```python
from build123d import *

# Parameters (mm, degrees)
EXTRUDE_THIN3_DEPTH     = 70
CUT_EXTRUDE1_DEPTH      = 76.511321578
CUT_EXTRUDE1_DEPTH_BACK = 76.511321578
SKETCH9_R               = 4.064
CUT_EXTRUDE2_DEPTH      = 2.54
LPATTERN1_COUNT         = 2
LPATTERN1_PITCH         = 12.7


# Read off the part's stored shape, not the designer's step: Mirror1
with BuildPart() as part:
    # Sketch6 → Extrude-Thin3 (new body)
    with BuildSketch(Plane.XY):
        Polygon((25.0952, 2.1336), (27.6352, 2.1336), (27.6352, 0), (-27.6352, 0), (-27.6352, 2.1336), (-25.0952, 2.1336), (-25.0952, 2.6416), (-28.1432, 2.6416), (-28.1432, -0.508), (28.1432, -0.508), (28.1432, 2.6416), (25.0952, 2.6416), align=None)
    extrude(amount=EXTRUDE_THIN3_DEPTH)

    # Sketch8 → Cut-Extrude1 (cut, two sides: drawn at the far end of the back side and taken through both)
    with BuildSketch(Plane.XZ.offset(0.508).offset(-CUT_EXTRUDE1_DEPTH_BACK)):
        with BuildLine():
            Line((5, 45), (5, 25))
            ThreePointArc((5, 25), (0, 20), (-5, 25))
            Line((-5, 25), (-5, 45))
            ThreePointArc((-5, 45), (0, 50), (5, 45))
        make_face()
    extrude(amount=CUT_EXTRUDE1_DEPTH + CUT_EXTRUDE1_DEPTH_BACK, mode=Mode.SUBTRACT)

    # Sketch9 → Cut-Extrude2 (cut)
    with BuildSketch(Plane.XZ.offset(0.508)):
        with Locations(Location((20.0152, 63.904, 0), (0, 0, 270))):
            Circle(SKETCH9_R)
    cut_extrude2 = extrude(amount=-CUT_EXTRUDE2_DEPTH, mode=Mode.SUBTRACT)

    # Sketch10 → Revolve1 (revolve)
    with BuildSketch(Plane(origin=(0, 0, 63.904), x_dir=(0, -1, 0), z_dir=(0, 0, 1)), mode=Mode.PRIVATE) as revolve1_sk:
        Polygon((0, 24.0792), (1.429807942, 21.6027), (2.016395815, 21.6027), (0, 25.0952), align=None)
    revolve1 = revolve(revolve1_sk.sketch.rotate(Axis((20.0152, 10.109887768, 63.904), (0, -1, 0)), 90), axis=Axis((20.0152, 10.109887768, 63.904), (0, -1, 0)))

    # LPattern1: Cut-Extrude2, Revolve1 ×2
    with Locations(*[(-i * LPATTERN1_PITCH, 0, 0) for i in range(1, LPATTERN1_COUNT)]):
        add(cut_extrude2, mode=Mode.SUBTRACT)
        add(revolve1)

    # Mirror1 outline → Mirror1 (revolve)
    with BuildSketch(Plane(origin=(20.0152, 0, 6.096), x_dir=(1, 0, 0), z_dir=(0, 0, 1))):
        Polygon((3.18411819, -0.508), (1.5875, -1.429807942), (1.5875, -2.016395815), (4.20011819, -0.508), align=None)
    revolve(axis=Axis((20.0152, 0, 6.096), (0, 1, 0)))

    # Mirror1 2 outline → Mirror1 2 (revolve)
    with BuildSketch(Plane(origin=(7.3152, 0, 6.096), x_dir=(1, 0, 0), z_dir=(0, 0, 1))):
        Polygon((3.18411819, -0.508), (1.5875, -1.429807942), (1.5875, -2.016395815), (4.20011819, -0.508), align=None)
    revolve(axis=Axis((7.3152, 0, 6.096), (0, 1, 0)))

    # Mirror1 3 outline → Mirror1 3 (revolve, cut)
    with BuildSketch(Plane(origin=(20.0152, 0, 6.096), x_dir=(1, 0, 0), z_dir=(0, 0, 1))):
        Polygon((3.18411819, -0.508), (4.064, 0), (0, 0), (0, -0.508), align=None)
    revolve(axis=Axis((20.0152, 0, 6.096), (0, 1, 0)), mode=Mode.SUBTRACT)

    # Mirror1 4 outline → Mirror1 4 (revolve, cut)
    with BuildSketch(Plane(origin=(7.3152, 0, 6.096), x_dir=(1, 0, 0), z_dir=(0, 0, 1))):
        Polygon((3.18411819, -0.508), (4.064, 0), (0, 0), (0, -0.508), align=None)
    revolve(axis=Axis((7.3152, 0, 6.096), (0, 1, 0)), mode=Mode.SUBTRACT)


solid = part.part
```
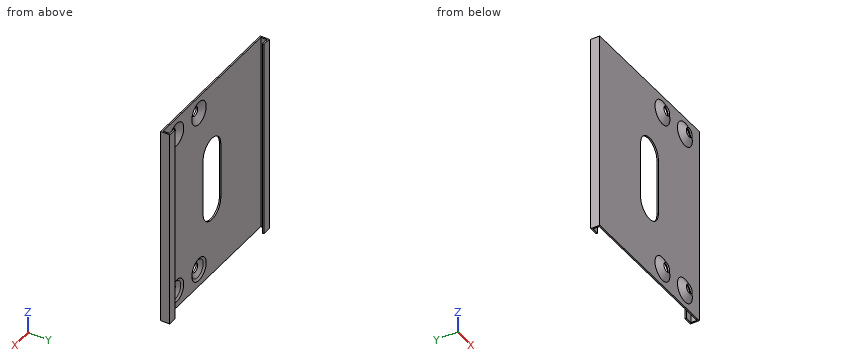
Geometry check sheet. Reference: the model listing, model coordinates, mm. Coordinates: 2 decimals unless noted, no trailing zeros. Write each loop counter-clockwise with the first axis right and the second up, starting at its lowest first coordinate (ties: lowest second). Pieces come first, ordered by that corner, then holes. Notation, with made-up numbers: (88.5, 54.5) -> (145.5, 54.5) arc R20 cw to (145.5, 58.5) -> close; hole circle Ø7 at (63.5, 21). An arc over 180 degrees is marked (long way). Use CSV: the item, a comma, the result in double quotes. Start each with the question number.
Item 1: Cross-section at A-A, the plane z = 41. Record the cut outline in (x, y), plus the area to 3 significant figures.
Item 2: Depth check by flat-ended pin: pin 1 Ø10 at (x, z) = (1, 26) entering from -Y; pin 2 Ø3.5 at (x, z) = (7.32, 63.9) entering from +Y; pin 3 Ø4 at (x, z) = (20.02, 63.9) entering from +Y. Enter the tip coordinate at first touch or a pass-through.
Item 3: Thickness scan on line 1 (X direction, y = 0.55, z = 3); line 2 (X direction, y = -0.1, z = 38); line 3 (Y direction, x = -26, z = 60.5). Record the ranges inside material, lowest first.
Item 4: Cross-section at B-B, the plane x = 0. Record the cut outline in (y, z), plus the area to 3 significant figures.
Item 5: Cross-section at D-D, the plane z = 18. Record the cut outline in (x, y).
Item 6: Cross-section at C-C, the plane y = 1.3. Record the cut outline in (x, z).
Answers:
1,outline,"(-28.14, -0.51) -> (-5, -0.51) -> (-5, 0) -> (-27.64, 0) -> (-27.64, 2.13) -> (-25.1, 2.13) -> (-25.1, 2.64) -> (-28.14, 2.64) -> close; (5, -0.51) -> (28.14, -0.51) -> (28.14, 2.64) -> (25.1, 2.64) -> (25.1, 2.13) -> (27.64, 2.13) -> (27.64, 0) -> (5, 0) -> close"
1,area,"28.8 mm^2"
2,pin 1,"y = -0.51"
2,pin 2,"y = -1.33"
2,pin 3,"y = -1.19"
3,line 1,"-28.14 to -27.64, 27.64 to 28.14"
3,line 2,"-28.14 to -5, 5 to 28.14"
3,line 3,"-0.51 to 0, 2.13 to 2.64"
4,outline,"(-0.51, 0) -> (0, 0) -> (0, 20) -> (-0.51, 20) -> close; (-0.51, 50) -> (0, 50) -> (0, 70) -> (-0.51, 70) -> close"
4,area,"20.3 mm^2"
5,outline,"(-28.14, -0.51) -> (28.14, -0.51) -> (28.14, 2.64) -> (25.1, 2.64) -> (25.1, 2.13) -> (27.64, 2.13) -> (27.64, 0) -> (-27.64, 0) -> (-27.64, 2.13) -> (-25.1, 2.13) -> (-25.1, 2.64) -> (-28.14, 2.64) -> close"
6,outline,"(-28.14, 0) -> (-27.64, 0) -> (-27.64, 70) -> (-28.14, 70) -> close; (27.64, 0) -> (28.14, 0) -> (28.14, 70) -> (27.64, 70) -> close"
